Input: part model. Units: mm. Frame: model coordinates. A direction names the side the tool comes from. Coordinates: 2 decimals unless noted, no trailing zeros. Write each loop counter-clockwise with the first axis right and the second up, starting at its lowest first coordinate (ties: lowest second). Pieces come first, ordered by that corner, then holes.
1) Set-up query: faces 4 (the flat face through (-3.159, -5.885, 0.521)), 5 (the flat face through (5.61, 3.61, 0.52)), 6 (the flat face through (-3.61, 5.61, 0.52)), 7 (the flat face through (-5.885, 3.159, 0.521)). Return all of +Z, -Z, +X, -X, +Y, -Y with unobstructed straight access to the full face (end or side cutting, diameter ignored); none if empty.
2) Section query A-A (y = -0.25). Output: boundary loops of the cut face in (x, z), then the cut area to 3 significant figures.
3) Line query: L1, parallel to Y at x = 6.5, z = 1; L2, parallel to Y at x = -0.5, z = 0.4; L3, parallel to X at y = -2, z = 1.6. Output: solid intervals per line, ascending.
4) Section query B-B (x = -2). Output: boundary loops of the cut face in (y, z), then the cut area to 3 significant figures.
5) Pin query (flat end, axial travel): pin 1 Ø0.6 at (y, z) = (-0.5, 0.5) entering from -X; pin 2 Ø1.5 at (y, z) = (5.5, 1.5) entering from -X. Return the tip coordinate at first contact, or that it passes through.
6) Draft query along Y for faces 1 (the flat face through (1.7, -6.45, 0.52)), 2 (the flat face through (2.382, 0, 1)), 3 (the flat face through (-5.17, 4.22, 0.52)). Return one class per face: pulls with the +Y half, pulls with the -Y half, needs draft (parallel to the pull), parting line crosses it, or undercut.
from build123d import *

# Parameters (mm, degrees)
F1_DEPTH = 2
F0_R     = 1
F2_DEPTH = 1


with BuildPart() as f1:
    # F0 (on Top) → F1 (new body)
    with BuildSketch(Plane.XY):
        with BuildLine():
            Line((6.32937, -0.741792), (7, 0))
            ThreePointArc((7, 0), (6.994284, 0.282817), (6.977147, 0.565173))
            Line((6.977147, 0.565173), (6.248815, 1.250397))
            Line((6.248815, 1.250397), (6.657396, 2.163119))
            ThreePointArc((6.657396, 2.163119), (6.564564, 2.430328), (6.461013, 2.693568))
            Line((6.461013, 2.693568), (5.556582, 3.120188))
            Line((5.556582, 3.120188), (5.663119, 4.114497))
            ThreePointArc((5.663119, 4.114497), (5.492259, 4.339941), (5.31243, 4.558299))
            Line((5.31243, 4.558299), (4.320432, 4.684553))
            Line((4.320432, 4.684553), (4.114497, 5.663119))
            ThreePointArc((4.114497, 5.663119), (3.882333, 5.824731), (3.64383, 5.976831))
            Line((3.64383, 5.976831), (2.661369, 5.790362))
            Line((2.661369, 5.790362), (2.163119, 6.657396))
            ThreePointArc((2.163119, 6.657396), (1.892377, 6.739355), (1.618546, 6.810309))
            Line((1.618546, 6.810309), (0.741792, 6.32937))
            Line((0.741792, 6.32937), (0, 7))
            ThreePointArc((0, 7), (-0.282817, 6.994284), (-0.565173, 6.977147))
            Line((-0.565173, 6.977147), (-1.250397, 6.248815))
            Line((-1.250397, 6.248815), (-2.163119, 6.657396))
            ThreePointArc((-2.163119, 6.657396), (-2.430328, 6.564564), (-2.693568, 6.461013))
            Line((-2.693568, 6.461013), (-3.120188, 5.556582))
            Line((-3.120188, 5.556582), (-4.114497, 5.663119))
            ThreePointArc((-4.114497, 5.663119), (-4.339941, 5.492259), (-4.558299, 5.31243))
            Line((-4.558299, 5.31243), (-4.684553, 4.320432))
            Line((-4.684553, 4.320432), (-5.663119, 4.114497))
            ThreePointArc((-5.663119, 4.114497), (-5.824731, 3.882333), (-5.976831, 3.64383))
            Line((-5.976831, 3.64383), (-5.790362, 2.661369))
            Line((-5.790362, 2.661369), (-6.657396, 2.163119))
            ThreePointArc((-6.657396, 2.163119), (-6.739355, 1.892377), (-6.810309, 1.618546))
            Line((-6.810309, 1.618546), (-6.32937, 0.741792))
            Line((-6.32937, 0.741792), (-7, 0))
            ThreePointArc((-7, 0), (-6.994284, -0.282817), (-6.977147, -0.565173))
            Line((-6.977147, -0.565173), (-6.248815, -1.250397))
            Line((-6.248815, -1.250397), (-6.657396, -2.163119))
            ThreePointArc((-6.657396, -2.163119), (-6.564564, -2.430328), (-6.461013, -2.693568))
            Line((-6.461013, -2.693568), (-5.556582, -3.120188))
            Line((-5.556582, -3.120188), (-5.663119, -4.114497))
            ThreePointArc((-5.663119, -4.114497), (-5.492259, -4.339941), (-5.31243, -4.558299))
            Line((-5.31243, -4.558299), (-4.320432, -4.684553))
            Line((-4.320432, -4.684553), (-4.114497, -5.663119))
            ThreePointArc((-4.114497, -5.663119), (-3.882333, -5.824731), (-3.64383, -5.976831))
            Line((-3.64383, -5.976831), (-2.661369, -5.790362))
            Line((-2.661369, -5.790362), (-2.163119, -6.657396))
            ThreePointArc((-2.163119, -6.657396), (-1.892377, -6.739355), (-1.618546, -6.810309))
            Line((-1.618546, -6.810309), (-0.741792, -6.32937))
            Line((-0.741792, -6.32937), (0, -7))
            ThreePointArc((0, -7), (0.282817, -6.994284), (0.565173, -6.977147))
            Line((0.565173, -6.977147), (1.250397, -6.248815))
            Line((1.250397, -6.248815), (2.163119, -6.657396))
            ThreePointArc((2.163119, -6.657396), (2.430328, -6.564564), (2.693568, -6.461013))
            Line((2.693568, -6.461013), (3.120188, -5.556582))
            Line((3.120188, -5.556582), (4.114497, -5.663119))
            ThreePointArc((4.114497, -5.663119), (4.339941, -5.492259), (4.558299, -5.31243))
            Line((4.558299, -5.31243), (4.684553, -4.320432))
            Line((4.684553, -4.320432), (5.663119, -4.114497))
            ThreePointArc((5.663119, -4.114497), (5.824731, -3.882333), (5.976831, -3.64383))
            Line((5.976831, -3.64383), (5.790362, -2.661369))
            Line((5.790362, -2.661369), (6.657396, -2.163119))
            ThreePointArc((6.657396, -2.163119), (6.739355, -1.892377), (6.810309, -1.618546))
            Line((6.810309, -1.618546), (6.32937, -0.741792))
        make_face()
        Polygon((2.38157, -1.375), (0, -2.75), (-2.38157, -1.375), (-2.38157, 1.375), (0, 2.75), (2.38157, 1.375), align=None, mode=Mode.SUBTRACT)
    extrude(amount=F1_DEPTH)

    # F0 (on Top) → F2 (join)
    with BuildSketch(Plane.XY):
        with BuildLine():
            Line((6.32937, -0.741792), (7, 0))
            ThreePointArc((7, 0), (6.994284, 0.282817), (6.977147, 0.565173))
            Line((6.977147, 0.565173), (6.248815, 1.250397))
            Line((6.248815, 1.250397), (6.657396, 2.163119))
            ThreePointArc((6.657396, 2.163119), (6.564564, 2.430328), (6.461013, 2.693568))
            Line((6.461013, 2.693568), (5.556582, 3.120188))
            Line((5.556582, 3.120188), (5.663119, 4.114497))
            ThreePointArc((5.663119, 4.114497), (5.492259, 4.339941), (5.31243, 4.558299))
            Line((5.31243, 4.558299), (4.320432, 4.684553))
            Line((4.320432, 4.684553), (4.114497, 5.663119))
            ThreePointArc((4.114497, 5.663119), (3.882333, 5.824731), (3.64383, 5.976831))
            Line((3.64383, 5.976831), (2.661369, 5.790362))
            Line((2.661369, 5.790362), (2.163119, 6.657396))
            ThreePointArc((2.163119, 6.657396), (1.892377, 6.739355), (1.618546, 6.810309))
            Line((1.618546, 6.810309), (0.741792, 6.32937))
            Line((0.741792, 6.32937), (0, 7))
            ThreePointArc((0, 7), (-0.282817, 6.994284), (-0.565173, 6.977147))
            Line((-0.565173, 6.977147), (-1.250397, 6.248815))
            Line((-1.250397, 6.248815), (-2.163119, 6.657396))
            ThreePointArc((-2.163119, 6.657396), (-2.430328, 6.564564), (-2.693568, 6.461013))
            Line((-2.693568, 6.461013), (-3.120188, 5.556582))
            Line((-3.120188, 5.556582), (-4.114497, 5.663119))
            ThreePointArc((-4.114497, 5.663119), (-4.339941, 5.492259), (-4.558299, 5.31243))
            Line((-4.558299, 5.31243), (-4.684553, 4.320432))
            Line((-4.684553, 4.320432), (-5.663119, 4.114497))
            ThreePointArc((-5.663119, 4.114497), (-5.824731, 3.882333), (-5.976831, 3.64383))
            Line((-5.976831, 3.64383), (-5.790362, 2.661369))
            Line((-5.790362, 2.661369), (-6.657396, 2.163119))
            ThreePointArc((-6.657396, 2.163119), (-6.739355, 1.892377), (-6.810309, 1.618546))
            Line((-6.810309, 1.618546), (-6.32937, 0.741792))
            Line((-6.32937, 0.741792), (-7, 0))
            ThreePointArc((-7, 0), (-6.994284, -0.282817), (-6.977147, -0.565173))
            Line((-6.977147, -0.565173), (-6.248815, -1.250397))
            Line((-6.248815, -1.250397), (-6.657396, -2.163119))
            ThreePointArc((-6.657396, -2.163119), (-6.564564, -2.430328), (-6.461013, -2.693568))
            Line((-6.461013, -2.693568), (-5.556582, -3.120188))
            Line((-5.556582, -3.120188), (-5.663119, -4.114497))
            ThreePointArc((-5.663119, -4.114497), (-5.492259, -4.339941), (-5.31243, -4.558299))
            Line((-5.31243, -4.558299), (-4.320432, -4.684553))
            Line((-4.320432, -4.684553), (-4.114497, -5.663119))
            ThreePointArc((-4.114497, -5.663119), (-3.882333, -5.824731), (-3.64383, -5.976831))
            Line((-3.64383, -5.976831), (-2.661369, -5.790362))
            Line((-2.661369, -5.790362), (-2.163119, -6.657396))
            ThreePointArc((-2.163119, -6.657396), (-1.892377, -6.739355), (-1.618546, -6.810309))
            Line((-1.618546, -6.810309), (-0.741792, -6.32937))
            Line((-0.741792, -6.32937), (0, -7))
            ThreePointArc((0, -7), (0.282817, -6.994284), (0.565173, -6.977147))
            Line((0.565173, -6.977147), (1.250397, -6.248815))
            Line((1.250397, -6.248815), (2.163119, -6.657396))
            ThreePointArc((2.163119, -6.657396), (2.430328, -6.564564), (2.693568, -6.461013))
            Line((2.693568, -6.461013), (3.120188, -5.556582))
            Line((3.120188, -5.556582), (4.114497, -5.663119))
            ThreePointArc((4.114497, -5.663119), (4.339941, -5.492259), (4.558299, -5.31243))
            Line((4.558299, -5.31243), (4.684553, -4.320432))
            Line((4.684553, -4.320432), (5.663119, -4.114497))
            ThreePointArc((5.663119, -4.114497), (5.824731, -3.882333), (5.976831, -3.64383))
            Line((5.976831, -3.64383), (5.790362, -2.661369))
            Line((5.790362, -2.661369), (6.657396, -2.163119))
            ThreePointArc((6.657396, -2.163119), (6.739355, -1.892377), (6.810309, -1.618546))
            Line((6.810309, -1.618546), (6.32937, -0.741792))
        make_face()
        Polygon((2.38157, -1.375), (0, -2.75), (-2.38157, -1.375), (-2.38157, 1.375), (0, 2.75), (2.38157, 1.375), align=None, mode=Mode.SUBTRACT)
        Polygon((-2.38157, -1.375), (0, -2.75), (2.38157, -1.375), (2.38157, 1.375), (0, 2.75), (-2.38157, 1.375), align=None)
        Circle(F0_R, mode=Mode.SUBTRACT)
    extrude(amount=-F2_DEPTH)


solid = f1.part
Answer:
1. face 4: +Z, -Z, -Y
1. face 5: +Z, -Z, +X
1. face 6: +Z, -Z, +Y
1. face 7: +Z, -Z, -X
2. outline: (-7, -1) - (-0.97, -1) - (-0.97, 0) - (-2.38, 0) - (-2.38, 2) - (-7, 2) - close; (0.97, -1) - (6.77, -1) - (6.77, 2) - (2.38, 2) - (2.38, 0) - (0.97, 0) - close
2. area: 29.8 mm2
3. L1: y = -2.25 to -1.05, -0.55 to 1.01, 1.81 to 2.6
3. L2: y = -6.55 to -2.46, 2.46 to 6.98
3. L3: x = -6.58 to -1.3, 1.3 to 6.71
4. outline: (-6.71, -1) - (6.58, -1) - (6.58, 2) - (1.6, 2) - (1.6, 0) - (-1.6, 0) - (-1.6, 2) - (-6.71, 2) - close
4. area: 33.5 mm2
5. pin 1: stops at x = -7
5. pin 2: stops at x = -4.63
6. face 1: pulls with the -Y half
6. face 2: undercut
6. face 3: pulls with the +Y half
